Work out the finished part from the listing and answer in its coordinate system (mm). Coordinates: 2 decimals unless noted, no trailing zeros. Loops run counter-clockwise (first coordinate to the right, second up) from the corner with the lowest first, then second, coordinate; pieces in that order, holes last. Notation, with made-up numbers: (24.5, 79) -> (58.5, 79) arc R27 cw to (58.5, 99) -> close; hole circle Ø5 at (22.25, 29.25). An arc over 180 degrees is marked (long way). Use a Markdown table: item, result. Add a question column.
```python
from build123d import *

# Parameters (mm, degrees)
BOSS_EXTRUDE1_DEPTH = 63
FILLET2_R           = 2


with BuildPart() as part:
    # Sketch1 → Boss-Extrude1 (new body)
    with BuildSketch(Plane(origin=(0, 0, 0), x_dir=(1, 0, 0), z_dir=(0, 1, 0))):
        with BuildLine():
            ThreePointArc((9.075357143, 2.44905956), (-9.4, 0), (9.075357143, -2.44905956))
            ThreePointArc((9.075357143, -2.44905956), (8.5, 0), (9.075357143, 2.44905956))
        make_face()
        with BuildLine():
            ThreePointArc((8.649642857, 2.486700312), (8.1, 0), (8.649642857, -2.486700312))
            ThreePointArc((8.649642857, -2.486700312), (-9, 0), (8.649642857, 2.486700312))
        make_face(mode=Mode.SUBTRACT)
    extrude(amount=BOSS_EXTRUDE1_DEPTH)

    # Fillet2
    fillet2_edges = [part.edges().sort_by_distance(p)[0] for p in [
        (9.075357143, 31.5, 2.44905956),
        (9.075357143, 31.5, -2.44905956),
    ]]
    fillet(fillet2_edges, radius=FILLET2_R)


solid = part.part
```
Item 1: Section A-A (x = 0) is taken. Determine the outline of the cut face in (y, z).
Item 2: Section B-B (z = 0) is taken. Determine the outline of the cut face in (x, y), then the cut area to 3 significant figures.
Item 3: Given pin 1 (1 mm diameter, centred on x = 3, y = 28.5, fed in from -Z); pin 2 (8 mm diameter, centred on x = -6, y = 12.5, fed in from +Z); pin 3 (3 mm diameter, centred on x = 3, y = 8.5, fed in from -Z); pin 4 (6 mm diameter, centred on x = -2, z = -5.5, fed in from -Y), each flat-ended and moving along its own axis, determine where each tip first touches the part or whether it passes through.
Item 4: Find the intervals of material crossed by probe 1 along Z at (x, y) = (0, 18); probe 2 along X at (y, z) = (53.5, 7.5); probe 3 along Z at (x, y) = (-5, 15), in increasing order.
Item 5: For a pull along X with two mould halves and no side action, classify faces 1 (the face through (8.5, 31.1, 0)), 2 (the face through (-9.393, 31.059, -0.367)), 3 (the face through (-9, 31, 0)) as +X half, -X half, draft (parallel to the pull), parting line (faces both ways), or undercut.
Output:
| question | item | result |
|---|---|---|
| 1 | outline | (0, -9.4) -> (63, -9.4) -> (63, -9) -> (0, -9) -> close; (0, 9) -> (63, 9) -> (63, 9.4) -> (0, 9.4) -> close |
| 2 | outline | (-9.4, 0) -> (-9, 0) -> (-9, 63) -> (-9.4, 63) -> close; (8.1, 0) -> (8.5, 0) -> (8.5, 63) -> (8.1, 63) -> close |
| 2 | area | 50.4 mm2 |
| 3 | pin 1 | stops at z = -9.06 |
| 3 | pin 2 | stops at z = 9.18 |
| 3 | pin 3 | stops at z = -9.28 |
| 3 | pin 4 | passes through |
| 4 | probe 1 | z = -9.4 to -9, 9 to 9.4 |
| 4 | probe 2 | x = -5.67 to -4.97, 4.97 to 5.67 |
| 4 | probe 3 | z = -7.96 to -7.48, 7.48 to 7.96 |
| 5 | face 1 | +X half |
| 5 | face 2 | parting line |
| 5 | face 3 | undercut |
